Design review of the part built by this model. Coordinates are the model's own, in mm. A direction names the side the tool comes from. Coordinates: 2 decimals unless noted, no trailing zeros. Order: outer loops, then holes, each group sorted by start corner. A loop starts at its lowest first (then second) coordinate and runs counter-clockwise, first axis right, second up. Notation, with made-up numbers: M -40,51.25 L -6,51.25 A24 ccw -6,87.25 Z; hole C 35.5,-24.5 d10. An arc over 180 degrees is marked long. Answer as a JSON object with one key per item and string values.
from build123d import *

# Parameters (mm, degrees)
SKETCH1_R           = 10
BOSS_EXTRUDE1_DEPTH = 2
SKETCH2_R           = 4.5
BOSS_EXTRUDE2_DEPTH = 2.5
SKETCH3_R           = 2.75
CUT_EXTRUDE1_DEPTH  = 3.5
SKETCH4_R           = 1.5
CUT_EXTRUDE2_DEPTH  = 2
SKETCH5_R           = 1.5
CUT_EXTRUDE3_DEPTH  = 3


with BuildPart() as part:
    # Sketch1 → Boss-Extrude1 (new body)
    with BuildSketch(Plane(origin=(0, 0, 0), x_dir=(1, 0, 0), z_dir=(0, 1, 0))):
        Circle(SKETCH1_R)
    extrude(amount=BOSS_EXTRUDE1_DEPTH)

    # Sketch2 → Boss-Extrude2 (add)
    with BuildSketch(Plane(origin=(0, 2, 0), x_dir=(1, 0, 0), z_dir=(0, 1, 0))):
        Circle(SKETCH2_R)
    extrude(amount=BOSS_EXTRUDE2_DEPTH)

    # Sketch3 → Cut-Extrude1 (cut)
    with BuildSketch(Plane(origin=(0, 4.5, 0), x_dir=(1, 0, 0), z_dir=(0, 1, 0))):
        Circle(SKETCH3_R)
    extrude(amount=-CUT_EXTRUDE1_DEPTH, mode=Mode.SUBTRACT)

    # Sketch4 → Cut-Extrude2 (cut, through all)
    with BuildSketch(Plane(origin=(0, 1, 0), x_dir=(1, 0, 0), z_dir=(0, 1, 0))):
        Circle(SKETCH4_R)
    extrude(amount=-CUT_EXTRUDE2_DEPTH, mode=Mode.SUBTRACT)

    # Sketch5 → Cut-Extrude3 (cut, through all)
    with BuildSketch(Plane(origin=(0, 2, 0), x_dir=(1, 0, 0), z_dir=(0, 1, 0))):
        with Locations((0, 7)):
            Circle(SKETCH5_R)
        with Locations((7, 0)):
            Circle(SKETCH5_R)
        with Locations((0, -7)):
            Circle(SKETCH5_R)
        with Locations((-7, 0)):
            Circle(SKETCH5_R)
    extrude(amount=-CUT_EXTRUDE3_DEPTH, mode=Mode.SUBTRACT)


solid = part.part
1) Add section B-B (z = 0). State the section outline as (x, y) points, and give its area (4 significant figures).
Taken from the geometry:
{"outline": "M -10,0 L -8.5,0 L -8.5,2 L -10,2 Z; M -5.5,0 L -1.5,0 L -1.5,1 L -2.75,1 L -2.75,4.5 L -4.5,4.5 L -4.5,2 L -5.5,2 Z; M 1.5,0 L 5.5,0 L 5.5,2 L 4.5,2 L 4.5,4.5 L 2.75,4.5 L 2.75,1 L 1.5,1 Z; M 8.5,0 L 10,0 L 10,2 L 8.5,2 Z", "area": "28.25 mm2"}
2) To check wall thickness, follow L1, parallel to Z at x = 0, y = 0.3; L2, parallel to Z at x = 0, y = 1.1. State the ranges of each line that lie inside material, in increasing order.
Taken from the geometry:
{"L1": "z = -10 to -8.5, -5.5 to -1.5, 1.5 to 5.5, 8.5 to 10", "L2": "z = -10 to -8.5, -5.5 to -2.75, 2.75 to 5.5, 8.5 to 10"}
3) Tool access review of faces 1 (the cylindrical face through (-0.596, 2.774, 2.685)), 2 (the flat face through (0, 4.5, 3)): name each direction out of +Z, -Z, +X, -X, +Y, -Y from which nothing blocks a thin tool from reaching the whole face with its end or side.
Taken from the geometry:
{"face 1": "+Y", "face 2": "+Z, -Z, +X, -X, +Y"}
4) Add section C-C (y = 0.4). State the section outline as (x, z) points, and give its area (3 significant figures).
Taken from the geometry:
{"outline": "C 0,0 d20; hole C -7,0 d3; hole C 0,-7 d3; hole C 0,0 d3; hole C 0,7 d3; hole C 7,0 d3", "area": "279 mm2"}
5) Add section A-A (x = 0). State the section outline as (y, z) points.
Taken from the geometry:
{"outline": "M 0,-10 L 2,-10 L 2,-8.5 L 0,-8.5 Z; M 0,-5.5 L 2,-5.5 L 2,-4.5 L 4.5,-4.5 L 4.5,-2.75 L 1,-2.75 L 1,-1.5 L 0,-1.5 Z; M 0,1.5 L 1,1.5 L 1,2.75 L 4.5,2.75 L 4.5,4.5 L 2,4.5 L 2,5.5 L 0,5.5 Z; M 0,8.5 L 2,8.5 L 2,10 L 0,10 Z"}
6) Add section D-D (x = 8). State the section outline as (y, z) points, and give its area (3 significant figures).
Taken from the geometry:
{"outline": "M 0,-6 L 2,-6 L 2,-1.12 L 0,-1.12 Z; M 0,1.12 L 2,1.12 L 2,6 L 0,6 Z", "area": "19.5 mm2"}
7) Mouldability with a two-part tool opening along X and no side actions: class faces 3 (the flat face through (0, 0, 2)), 4 (the cylindrical face through (-0.59, 3.23, -4.46)), 5 (the cylindrical face through (-0.325, 1.014, 8.464)), 6 (the cylindrical face through (-1.5, 0.51, -0.07)) as released by +X, released by -X, zero draft, split by the parting line, or undercut.
Taken from the geometry:
{"face 3": "zero draft", "face 4": "split by the parting line", "face 5": "undercut", "face 6": "undercut"}
8) Insertion check: pin 1 Ø4 at (x, z) = (-2, 7.5) entering from +Y; pin 2 Ø4.5 at (x, z) = (0, 0) entering from +Y; pin 3 Ø1.5 at (x, y) = (-5.5, 2.5) entering from +Z. Each pin has a flat end and moves straight along its axis. Give the tip position at first contact, or say it passes through.
Taken from the geometry:
{"pin 1": "stops at y = 2", "pin 2": "stops at y = 1", "pin 3": "stops at z = 8.69"}
